from build123d import *

# Parameters (mm, degrees)
SKETCH1_W               = 57.15
SKETCH1_H               = 31.75
BOSS_EXTRUDE1_DEPTH     = 1.651
SKETCH2_R               = 1.4732
MOUNT_HOLES_DEPTH       = 2.651
SKETCH3_W               = 23.114
SKETCH3_H               = 6.604
BOSS_EXTRUDE2_DEPTH     = 8.636
CUT_EXTRUDE1_DEPTH      = 23.114
SKETCH5_W               = 9.906
SKETCH5_H               = 9.906
LARGE_BOTTOM_CHIP_DEPTH = 1.524
SKETCH8_R               = 5.9055
BUZZER_DEPTH            = 5.08
SKETCH9_W               = 7.62
SKETCH9_H               = 5.842
USB_CONNECTOR_DEPTH     = 2.54


with BuildPart() as part:
    # Sketch1 → Boss-Extrude1 (new body)
    with BuildSketch(Plane.XY):
        Rectangle(SKETCH1_W, SKETCH1_H)
    extrude(amount=BOSS_EXTRUDE1_DEPTH)

    # Sketch2 → Mount-Holes (cut, through all)
    with BuildSketch(Plane.XY.offset(1.651)):
        with Locations((25.4, -12.7)):
            Circle(SKETCH2_R)
        with Locations((25.4, 12.7)):
            Circle(SKETCH2_R)
        with Locations((-25.4, 12.7)):
            Circle(SKETCH2_R)
        with Locations((-25.4, -12.7)):
            Circle(SKETCH2_R)
    extrude(amount=-MOUNT_HOLES_DEPTH, mode=Mode.SUBTRACT)

    # Sketch3 → Boss-Extrude2 (add)
    with BuildSketch(Plane.XY.offset(1.651)):
        with Locations((-11.938, -3.556)):
            Rectangle(SKETCH3_W, SKETCH3_H)
    boss_extrude2 = extrude(amount=BOSS_EXTRUDE2_DEPTH)

    # Sketch4 → Cut-Extrude1 (cut)
    with BuildSketch(Plane.ZY.offset(23.495)):
        Polygon((6.223, -6.858), (10.287, -5.334), (10.287, -6.858), align=None)
        Polygon((10.287, -0.254), (10.287, -1.778), (6.223, -0.254), align=None)
    cut_extrude1 = extrude(amount=-CUT_EXTRUDE1_DEPTH, mode=Mode.SUBTRACT)

    # Mirror1: Boss-Extrude2, Cut-Extrude1 across plane
    add(boss_extrude2.mirror(Plane.ZX))
    add(cut_extrude1.mirror(Plane.ZX), mode=Mode.SUBTRACT)

    # Sketch5 → Large bottom chip (add)
    with BuildSketch(Plane(origin=(0, 0, 0), x_dir=(-1, 0, 0), z_dir=(0, 0, -1))):
        with Locations((-15.24, 0)):
            Rectangle(SKETCH5_W, SKETCH5_H)
    extrude(amount=LARGE_BOTTOM_CHIP_DEPTH)

    # Sketch8 → Buzzer (add)
    with BuildSketch(Plane.XY.offset(1.651)):
        with Locations((5.969, 0)):
            Circle(SKETCH8_R)
    extrude(amount=BUZZER_DEPTH)

    # Sketch9 → USB Connector (add)
    with BuildSketch(Plane(origin=(0, 0, 0), x_dir=(-1, 0, 0), z_dir=(0, 0, -1))):
        with Locations((-0.635, -12.827)):
            Rectangle(SKETCH9_W, SKETCH9_H)
    extrude(amount=USB_CONNECTOR_DEPTH)


solid = part.part
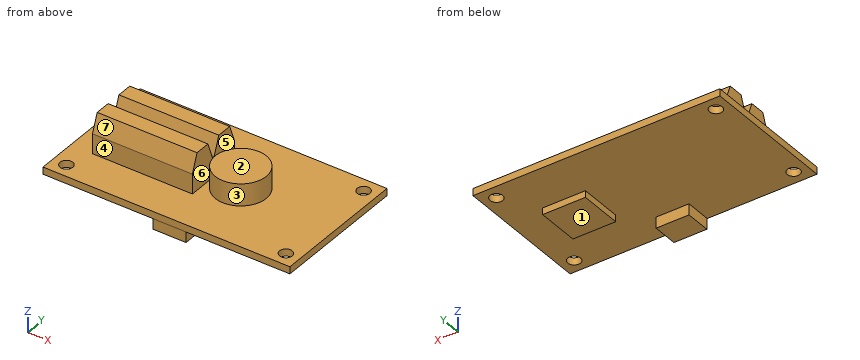
The listing builds one solid part. Answer for the finished solid, in the listing's coordinates (mm). Face numbers are marked on the shaded views. A direction names the side the tool comes from. Coordinates: 2 decimals unless noted, no trailing zeros. Order: outer loops, then holes, each group sorted by start corner. A loop starts at its lowest first (then second) coordinate and runs counter-clockwise, first axis right, second up. Notation, with made-up numbers: (54, 25) -> (75, 25) arc R25 cw to (75, 49) -> close; hole circle Ø6 at (-39.75, -7). An arc over 180 degrees is marked (long way). Answer in a Markdown table with one row per item. Add a question column.
Item 1: Find section D-D (x = -9.5). Write down the section's boundary in (y, z) (3 decimals), then the cut area to 3 significant figures.
Item 2: Find section A-A (x = -25.4). Write down the section's boundary in (y, z) (3 decimals).
Item 3: Find the intervals of material crossed by L1, parallel to Y at x = -25.4, z = 0.6 (3 decimals); L2, parallel to Y at x = -7.5, z = 5; L3, parallel to Z at x = 17.5, y = 10, in increasing order. Write a range as from..to.
Item 4: Find section C-C (z = 3.5). Write down the section's boundary in (x, y) (1 decimal), then the cut area to 3 significant figures.
Item 5: Find section B-B (y = -12.7). Write down the section's boundary in (x, z) (3 decimals), then the cut area to 3 significant figures.
Item 6: Which of the six approach directions +Z, -Z, +X, -X, +Y, -Y give full straight-line access (tool end or side, diameter ignored) to the marked faces 1, 2, 3 and 4?
Item 7: Determine the mould class of the marked faces 5, 6 and 7 for opening direction X: +X half, -X half, draft (parallel to the pull), parting line (faces both ways), or undercut.
Item 8: Each of these flat-tipped pins is pushed along its axis until it touches: P1, Ø2.5, axis at x = -13, z = 3.5, coming from the +Y side; P2, Ø1, axis at y = 1.5, z = 5, coming from the +X side; P3, Ø0.8, axis at x = 14.5, z = -0.5, coming from the +Y side. Where does it stop, or does it pass through?
Result set:
| question | item | result |
|---|---|---|
| 1 | outline | (-15.875, 0) -> (15.875, 0) -> (15.875, 1.651) -> (6.858, 1.651) -> (6.858, 6.223) -> (5.334, 10.287) -> (1.778, 10.287) -> (0.254, 6.223) -> (0.254, 1.651) -> (-0.254, 1.651) -> (-0.254, 6.223) -> (-1.778, 10.287) -> (-5.334, 10.287) -> (-6.858, 6.223) -> (-6.858, 1.651) -> (-15.875, 1.651) -> close |
| 1 | area | 154 mm² |
| 2 | outline | (-15.875, 0) -> (-14.173, 0) -> (-14.173, 1.651) -> (-15.875, 1.651) -> close; (-11.227, 0) -> (11.227, 0) -> (11.227, 1.651) -> (-11.227, 1.651) -> close; (14.173, 0) -> (15.875, 0) -> (15.875, 1.651) -> (14.173, 1.651) -> close |
| 3 | L1 | y = -15.875..-14.173, -11.227..11.227, 14.173..15.875 |
| 3 | L2 | y = -6.86..-0.25, 0.25..6.86 |
| 3 | L3 | z = 0..1.65 |
| 4 | outline | (-23.5, -6.9) -> (-0.4, -6.9) -> (-0.4, -0.3) -> (-23.5, -0.3) -> close; (-23.5, 0.3) -> (-0.4, 0.3) -> (-0.4, 6.9) -> (-23.5, 6.9) -> close; circle Ø11.8 at (6, 0) |
| 4 | area | 415 mm² |
| 5 | outline | (-28.575, 0) -> (-26.873, 0) -> (-26.873, 1.651) -> (-28.575, 1.651) -> close; (-23.927, 0) -> (-3.175, 0) -> (-3.175, -2.54) -> (4.445, -2.54) -> (4.445, 0) -> (23.927, 0) -> (23.927, 1.651) -> (-23.927, 1.651) -> close; (26.873, 0) -> (28.575, 0) -> (28.575, 1.651) -> (26.873, 1.651) -> close |
| 5 | area | 104 mm² |
| 6 | face 1 | -Z, +X, -X, +Y, -Y |
| 6 | face 2 | +Z, +X, +Y, -Y |
| 6 | face 3 | +Z |
| 6 | face 4 | +Z, +X, -X, -Y |
| 7 | face 5 | undercut |
| 7 | face 6 | undercut |
| 7 | face 7 | draft |
| 8 | P1 | stops at y = 6.86 |
| 8 | P2 | stops at x = 11.79 |
| 8 | P3 | stops at y = 4.95 |
